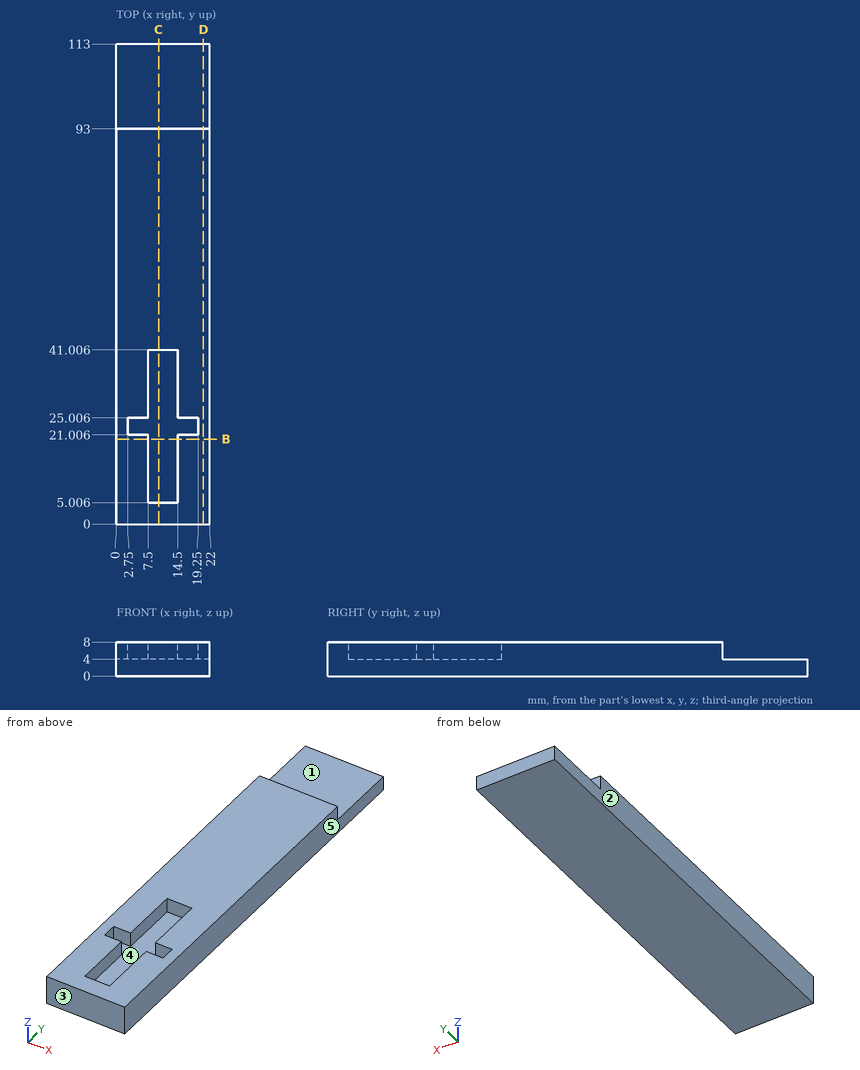
Geometry: see drawing. Coordinates: mm, zero at the bounding-box minimum. A direction names the side the tool comes from. Give positions to 0.01 mm unless a question says otherwise; leave off trailing zeros. Write each loop counter-clockwise with the first axis right and the second up, starting at its lowest first coordinate (ties: lowest second). Pieces come first, ordered by that corner, then holes. Notation, with made-up numbers: M 71,19.5 L 100,19.5 A27 cw 100,51.5 Z; hole C 49,-27.5 d4. An arc over 180 degrees is marked long. Answer in a Markdown table with one row per item. Add a question column.
(1) Mould query, pull axis X, two halves, no side actions, for the marked faces 3, 4 and 5. Classes: +X half, -X half, draft (parallel to the pull), parting line (faces both ways), or undercut.
(2) Ray query, line 1 (Y direction, x = 18.5, z = 4.25) (1 decimal); line 2 (Y direction, x = 10.25, z = 7.5) (1 decimal); line 3 (X direction, y = 24.5, z = 6.5). Return the intervals inside material, ascending.
(3) Reachability of the marked faces 1 and 2 from +Z, -Z, +X, -X, +Y, -Y: full face, straight path, thin tool, end or side. Return the list, or none.
(4) Section B-B on y = 20. Return loops of the section in (x, z).
(5) Section D-D on x = 20.5. Return loops of the section in (y, z), and give its area (3 significant figures).
(6) Section C-C on x = 10. Return loops of the section in (y, z) (1 decimal).
(7) First-contact query: pin 1 (1 mm diameter, centred on y = 94, z = 6.5, fed in from +X); pin 2 (1.2 mm diameter, centred on x = 11.5, z = 7, fed in from +Y). Flat tips, straight axial feed; report the tip coordinate or a pass-through.
Result set:
| question | item | result |
|---|---|---|
| 1 | face 3 | draft |
| 1 | face 4 | undercut |
| 1 | face 5 | +X half |
| 2 | line 1 | y = 0 to 21, 25 to 93 |
| 2 | line 2 | y = 0 to 5, 41 to 93 |
| 2 | line 3 | x = 0 to 2.75, 19.25 to 22 |
| 3 | face 1 | +Z, +X, -X, +Y |
| 3 | face 2 | +Z, -Z, -X, +Y, -Y |
| 4 | outline | M 0,0 L 22,0 L 22,8 L 14.5,8 L 14.5,4 L 7.5,4 L 7.5,8 L 0,8 Z |
| 5 | outline | M 0,0 L 113,0 L 113,4 L 93,4 L 93,8 L 0,8 Z |
| 5 | area | 824 mm^2 |
| 6 | outline | M 0,0 L 113,0 L 113,4 L 93,4 L 93,8 L 41,8 L 41,4 L 5,4 L 5,8 L 0,8 Z |
| 7 | pin 1 | passes through |
| 7 | pin 2 | stops at y = 93 |
